from build123d import *

# Parameters (mm, degrees)
F0_R     = 12.7
F1_DEPTH = 57.15
F2_DEPTH = 44.45
F3_R     = 5.08
F4_DEPTH = 13.7612578348


with BuildPart() as f1:
    # F0 (on Front) → F1 (new body)
    with BuildSketch(Plane.XZ):
        with BuildLine():
            Line((-31.75, -8.89), (-31.75, -21.59))
            Line((-31.75, -21.59), (31.75, -21.59))
            Line((31.75, -21.59), (31.75, -8.89))
            Line((31.75, -8.89), (12.7, -8.89))
            Line((12.7, -8.89), (12.7, 0))
            Line((12.7, 0), (63.5, 0))
            Line((63.5, 0), (63.5, 12.7))
            Line((63.5, 12.7), (47.625, 12.7))
            Line((47.625, 12.7), (21.0934256055, 52.2501730104))
            ThreePointArc((21.0934256055, 52.2501730104), (11.9529411765, 60.5117647059), (0, 63.5))
            ThreePointArc((0, 63.5), (-11.9529411765, 60.5117647059), (-21.0934256055, 52.2501730104))
            Line((-21.0934256055, 52.2501730104), (-47.625, 12.7))
            Line((-47.625, 12.7), (-63.5, 12.7))
            Line((-63.5, 12.7), (-63.5, 0))
            Line((-63.5, 0), (-12.7, 0))
            Line((-12.7, 0), (-12.7, -8.89))
            Line((-12.7, -8.89), (-31.75, -8.89))
        make_face()
        with Locations((0, 38.1)):
            Circle(F0_R, mode=Mode.SUBTRACT)
        with BuildLine():
            Line((-63.5, 63.5), (-63.5, 12.7))
            Line((-63.5, 12.7), (-47.625, 12.7))
            Line((-47.625, 12.7), (-21.0934256055, 52.2501730104))
            ThreePointArc((-21.0934256055, 52.2501730104), (-11.9529411765, 60.5117647059), (0, 63.5))
            Line((0, 63.5), (-63.5, 63.5))
        make_face()
        with BuildLine():
            Line((47.625, 12.7), (63.5, 12.7))
            Line((63.5, 12.7), (63.5, 63.5))
            Line((63.5, 63.5), (0, 63.5))
            ThreePointArc((0, 63.5), (11.9529411765, 60.5117647059), (21.0934256055, 52.2501730104))
            Line((21.0934256055, 52.2501730104), (47.625, 12.7))
        make_face()
    extrude(amount=-F1_DEPTH)

    # F0 (on Front) → F2 (cut)
    with BuildSketch(Plane.XZ):
        with BuildLine():
            Line((-63.5, 63.5), (-63.5, 12.7))
            Line((-63.5, 12.7), (-47.625, 12.7))
            Line((-47.625, 12.7), (-21.0934256055, 52.2501730104))
            ThreePointArc((-21.0934256055, 52.2501730104), (-11.9529411765, 60.5117647059), (0, 63.5))
            Line((0, 63.5), (-63.5, 63.5))
        make_face()
        with BuildLine():
            Line((47.625, 12.7), (63.5, 12.7))
            Line((63.5, 12.7), (63.5, 63.5))
            Line((63.5, 63.5), (0, 63.5))
            ThreePointArc((0, 63.5), (11.9529411765, 60.5117647059), (21.0934256055, 52.2501730104))
            Line((21.0934256055, 52.2501730104), (47.625, 12.7))
        make_face()
    extrude(amount=-F2_DEPTH, mode=Mode.SUBTRACT)

    # F3 (on face) → F4 (cut, through all)
    with BuildSketch(Plane.XY.offset(63.5)):
        with Locations((0, 22.225)):
            Circle(F3_R)
    extrude(amount=-F4_DEPTH, mode=Mode.SUBTRACT)


solid = f1.part
Can you work these out from the model? Positions are in its coordinate system, mm. A direction names the side the tool comes from. Coordinates: 2 decimals unless noted, no trailing zeros. Write each loop counter-clockwise with the first axis right and the second up, starting at its lowest first coordinate (ties: lowest second). Pieces come first, ordered by that corner, then holes.
Q1. Imagine slicing it at D-D, the plane z = 22. List the corners of the cut face in (x, y) for me, plus the area to 3 significant figures.
Results found:
outline: (-63.5, 44.45) - (-41.39, 44.45) - (-41.39, 0) - (41.39, 0) - (41.39, 44.45) - (63.5, 44.45) - (63.5, 57.15) - (-63.5, 57.15) - close
area: 5,290 mm2
Q2. Imagine slicing it at A-A, the plane z = 38.1. List the corners of the cut face in (x, y) for me, plus the area to 3 significant figures.
Results found:
outline: (-63.5, 44.45) - (-30.59, 44.45) - (-30.59, 0) - (-12.7, 0) - (-12.7, 57.15) - (-63.5, 57.15) - close; (12.7, 0) - (30.59, 0) - (30.59, 44.45) - (63.5, 44.45) - (63.5, 57.15) - (12.7, 57.15) - close
area: 2,880 mm2
Q3. Which directions (+Z, -Z, +X, -X, +Y, -Y) give clear straight access to the entire face, cutting with the end or side of a thin tool? Please do faces 1 (the face through (45, 44.45, 44)), 2 (the face through (22, 28, -8.89)), 3 (the face through (-34.545, 21.914, 32.198)), 4 (the face through (4.7, 20.3, 56.7)), 5 (the face through (-12.7, 28, -4)).
Results found:
face 1: +Z, +X, -Y
face 2: +X, +Y, -Y
face 3: +Z, -X, -Y
face 4: +Z
face 5: -X, +Y, -Y
Q4. Please list where these lines run through material, in increasing order: L1, parallel to Z at x = 0, y = 30; L2, parallel to Z at x = -31, y = 48; L3, parallel to Y at x = 0, z = 56.5 (3 decimals).
Results found:
L1: z = -21.59 to 25.4, 50.8 to 63.5
L2: z = -21.59 to -8.89, 0 to 63.5
L3: y = 0 to 17.145, 27.305 to 57.15
Q5. Imagine slicing it at C-C, the plane x = 17.5. List the corners of the cut face in (y, z) for me, plus the area to 3 significant figures.
Results found:
outline: (0, -21.59) - (57.15, -21.59) - (57.15, -8.89) - (0, -8.89) - close; (0, 0) - (57.15, 0) - (57.15, 63.5) - (44.45, 63.5) - (44.45, 56.51) - (0, 56.51) - close
area: 4,040 mm2
Q6. For P1, Ø17.5, axis at x = 58.5, y = 13.5, coming from the +Z side; P2, Ø4, axis at y = 40.5, z = -18, coming from the +X side; P3, Ø14, axis at y = 40, z = -16, coming from the -X side, each with a flat end and sliding along its axis, tell me the tip position at first contact or that it passes through.
Results found:
P1: stops at z = 12.7
P2: stops at x = 31.75
P3: stops at x = -31.75
Q7. If we mould it in two halves opening along Z, with no side actions, what happens to faces 6 (the face through (-63.5, 47, 18)), 7 (the face through (-56, 22, 12.7)), 8 (the face through (-22, 28, -8.89))? For each: +Z half, -Z half, draft (parallel to the pull), parting line (faces both ways), or undercut.
Results found:
face 6: draft
face 7: +Z half
face 8: undercut
Q8. Imagine slicing it at B-B, the plane y = 35. List the corners of the cut face in (x, z) for me (3 decimals), plus the area to 3 significant figures.
Results found:
outline: (-63.5, 0) - (-12.7, 0) - (-12.7, -8.89) - (-31.75, -8.89) - (-31.75, -21.59) - (31.75, -21.59) - (31.75, -8.89) - (12.7, -8.89) - (12.7, 0) - (63.5, 0) - (63.5, 12.7) - (47.625, 12.7) - (21.093, 52.25) arc R25.4 ccw to (-21.093, 52.25) - (-47.625, 12.7) - (-63.5, 12.7) - close; hole circle Ø25.4 at (0, 38.1)
area: 5,190 mm2
